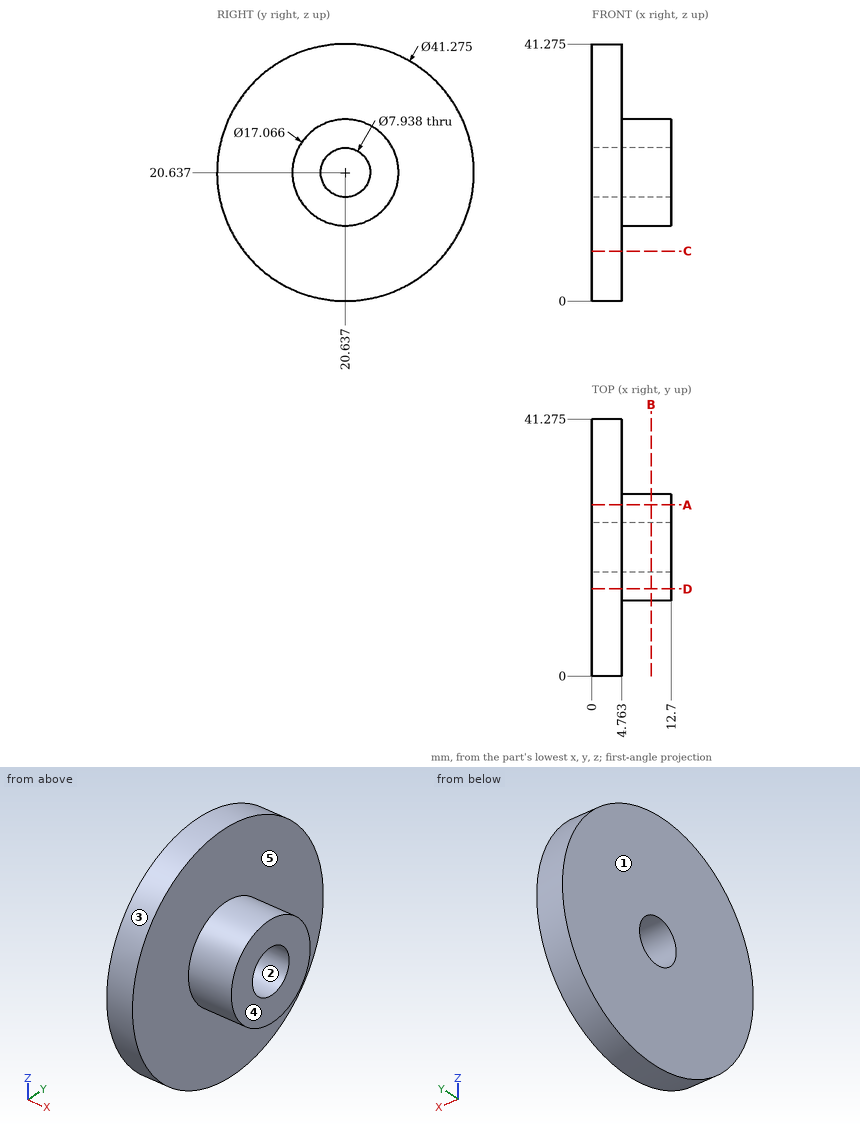
Verification items for this drawing (mm, ordinates from the low corner). A direction names the side the tool comes from. Give positions to 0.01 mm unless a question says otherwise; leave off trailing zeros. Write each loop counter-clockwise with the first axis right and the second up, starting at its lowest first coordinate (ties: lowest second). Pieces come first, ordered by that corner, then holes. Notation, with made-up numbers: (57, 56.25) - (88, 56.25) arc R31 cw to (88, 81.25) - close; hole circle Ø2 at (-19.75, -16). An arc over 180 degrees is marked (long way). Answer as CSV lines item,"result". Start each with the question number.
1. Sectioned sample at A-A (y = 27.5). Record the boundary of the cut face in (x, z) (1 decimal).
2. Depth check by flat-ended pin: pin 1 (1.5 mm diameter, centred on x = 1.5, z = 19, fed in from +Y); pin 2 (4 mm diameter, centred on y = 32.5, z = 8.5, fed in from +X); pin 3 (1 mm diameter, centred on x = 1.5, y = 23, fed in from +Z). Enter the tip coordinate at first touch or a pass-through.
3. Sectioned sample at C-C (z = 8). Record the boundary of the cut face in (x, y), then the cut area to 3 significant figures.
4. Thickness scan on line 1 (X direction, y = 26.5, z = 32.5); line 2 (Z direction, x = 1.5, y = 18) (1 decimal); line 3 (Y direction, x = 1.5, z = 25.5) (1 decimal). Record the ranges inside material, lowest first.
5. Sectioned sample at B-B (x = 9.5). Record the boundary of the cut face in (y, z) (1 decimal), then the cut area to 3 significant figures.
6. Draft check along Z on the marked faces 1, 2 and 3. Enter one of: pulls with the +Z half, pulls with the -Z half, needs draft (parallel to the pull), parting line crosses it, or undercut.
7. Set-up check for the marked faces 4 and 5: record each of +Z, -Z, +X, -X, +Y, -Y from which the full face is reachable in a straight line by a thin tool's end or side.
8. Sectioned sample at D-D (y = 14). Record the boundary of the cut face in (x, z) (1 decimal), then the cut area to 3 significant figures.
Derived:
1,outline,"(0, 1.2) - (4.8, 1.2) - (4.8, 15.6) - (12.7, 15.6) - (12.7, 25.7) - (4.8, 25.7) - (4.8, 40.1) - (0, 40.1) - close"
2,pin 1,"y = 41.26"
2,pin 2,"x = 4.76"
2,pin 3,"z = 41.19"
3,outline,"(0, 4.32) - (4.76, 4.32) - (4.76, 36.95) - (0, 36.95) - close"
3,area,"155 mm²"
4,line 1,"0 to 4.76"
4,line 2,"0.2 to 17.7, 23.6 to 41.1"
4,line 3,"0.6 to 40.7"
5,outline,"circle Ø17.1 at (20.6, 20.6); hole circle Ø7.9 at (20.6, 20.6)"
5,area,"179 mm²"
6,face 1,"needs draft"
6,face 2,"undercut"
6,face 3,"parting line crosses it"
7,face 4,"+Z, -Z, +X, +Y, -Y"
7,face 5,"+X"
8,outline,"(0, 1.1) - (4.8, 1.1) - (4.8, 15.3) - (12.7, 15.3) - (12.7, 26) - (4.8, 26) - (4.8, 40.2) - (0, 40.2) - close"
8,area,"271 mm²"
